Part model, mm, in its own coordinate system. A direction names the side the tool comes from. Coordinates: 2 decimals unless noted, no trailing zeros. Order: outer loops, then holes, each group sorted by start corner. A loop starts at its lowest first (then second) coordinate and runs counter-clockwise, first axis right, second up. Notation, with made-up numbers: (18.25, -23) - (59.25, -23) arc R12 ccw to (59.25, -12) - close; hole circle Ø3 at (16.25, 41.25). An arc over 180 degrees is marked (long way). Use a Markdown table: item, result. Add a question column.
1) Saw through at D-D on y = -12.5. List the corners of the cut face in (x, z).
2) Wall check: L1, parallel to Y at x = 0, z = 5.4; L2, parallel to Y at x = 0, z = 12; L3, parallel to Z at x = 1.5, y = 9.5. Give the ranges that are in metal, low to high. Write a range as [from, to].
3) Two-plate mould, pull along Z, no slides. Class faces 1 (the face through (-3, 7, 20)), 2 (the face through (8.873, -0.192, 13.098)), 3 (the face through (0, -9, 2)): +Z half, -Z half, draft (parallel to the pull), parting line (faces both ways), or undercut.
4) Saw through at B-B on x = 6. List the corners of the cut face in (y, z).
5) Saw through at A-A on y = 0. List the corners of the cut face in (x, z) (3 decimals), then the cut area to 4 significant figures.
6) Saw through at C-C on z = 3. List the corners of the cut face in (x, y), then the cut area to 3 significant figures.
7) Tool access for faces 4 (the face through (-2.981, -13.423, 4.986)), 5 (the face through (-8.873, 0.192, 13.098)), 6 (the face through (6.466, -2.681, 9.154)), 7 (the face through (9, 0, 4)): list every direction of +Z, -Z, +X, -X, +Y, -Y with a clear straight run to the whole face (end or side of a thin tool).
8) Drop flat-ended pins along their axis: P1, Ø12, axis at y = -13.5, z = 16.5, coming from the +X side; P2, Ø22, axis at x = 1, y = -6.5, coming from the +Z side; P3, Ø3, axis at y = -1, z = 7, coming from the +X side; P4, Ø6, axis at y = -9, z = 2.5, coming from the -X side. Give the stop position or say it passes through.
```python
from build123d import *

# Parameters (mm, degrees)
SKETCH1_R           = 13.75
BOSS_EXTRUDE1_DEPTH = 2
SKETCH2_R           = 8.5
BOSS_EXTRUDE2_DEPTH = 6
BOSS_EXTRUDE3_START = 4
SKETCH3_R           = 13.75
BOSS_EXTRUDE3_DEPTH = 2
SKETCH5_R           = 7
CUT_EXTRUDE2_DEPTH  = 37.5
BOSS_EXTRUDE4_START = 20
SKETCH6_R           = 8.875
SKETCH6_R_2         = 7
BOSS_EXTRUDE4_DEPTH = 14
CUT_EXTRUDE3_START  = 4
SKETCH9_R           = 0.25
CUT_EXTRUDE3_DEPTH  = 24.894892006
SKETCH10_R          = 19
BOSS_EXTRUDE5_DEPTH = 2
SKETCH11_R          = 7
CUT_EXTRUDE4_DEPTH  = 2
BOSS_EXTRUDE6_START = 2
SKETCH12_R          = 19
SKETCH12_R_2        = 17
BOSS_EXTRUDE6_DEPTH = 2


with BuildPart() as part:
    # Sketch1 → Boss-Extrude1 (new body)
    with BuildSketch(Plane.XY):
        Circle(SKETCH1_R)
    extrude(amount=BOSS_EXTRUDE1_DEPTH)

    # Sketch2 → Boss-Extrude2 (add)
    with BuildSketch(Plane.XY):
        Circle(SKETCH2_R)
    extrude(amount=BOSS_EXTRUDE2_DEPTH)

    # Sketch3 → Boss-Extrude3 (add)
    with BuildSketch(Plane.XY.offset(BOSS_EXTRUDE3_START)):
        Circle(SKETCH3_R)
    extrude(amount=BOSS_EXTRUDE3_DEPTH)

    # Sketch5 → Cut-Extrude2 (cut, symmetric)
    with BuildSketch(Plane.XY):
        Circle(SKETCH5_R)
    extrude(amount=CUT_EXTRUDE2_DEPTH, both=True, mode=Mode.SUBTRACT)

    # Sketch6 → Boss-Extrude4 (add)
    with BuildSketch(Plane.XY.offset(BOSS_EXTRUDE4_START)):
        Circle(SKETCH6_R)
        Circle(SKETCH6_R_2, mode=Mode.SUBTRACT)
    extrude(amount=-BOSS_EXTRUDE4_DEPTH)

    # Sketch9 → Cut-Extrude3 (cut, through all)
    with BuildSketch(Plane.XY.offset(CUT_EXTRUDE3_START)):
        with Locations((0, 9.75)):
            Circle(SKETCH9_R)
        with Locations((0, -9.75)):
            Circle(SKETCH9_R)
        with Locations(Location((0, 8.75, 0), (0, 0, 150.706355545))):
            Circle(SKETCH9_R)
        with Locations(Location((0, -8.75, 0), (0, 0, 209.293644455))):
            Circle(SKETCH9_R)
    extrude(amount=CUT_EXTRUDE3_DEPTH, mode=Mode.SUBTRACT)

    # Sketch10 → Boss-Extrude5 (add)
    with BuildSketch(Plane.XY):
        Circle(SKETCH10_R)
    extrude(amount=-BOSS_EXTRUDE5_DEPTH)

    # Sketch11 → Cut-Extrude4 (cut)
    with BuildSketch(Plane.XY):
        Circle(SKETCH11_R)
    extrude(amount=-CUT_EXTRUDE4_DEPTH, mode=Mode.SUBTRACT)

    # Sketch12 → Boss-Extrude6 (add)
    with BuildSketch(Plane.XY.offset(BOSS_EXTRUDE6_START)):
        Circle(SKETCH12_R)
        Circle(SKETCH12_R_2, mode=Mode.SUBTRACT)
    extrude(amount=-BOSS_EXTRUDE6_DEPTH)


solid = part.part
```
Results are:
| question | item | result |
|---|---|---|
| 1 | outline | (-14.31, -2) - (14.31, -2) - (14.31, 2) - (11.52, 2) - (11.52, 0) - (5.73, 0) - (5.73, 2) - (-5.73, 2) - (-5.73, 0) - (-11.52, 0) - (-11.52, 2) - (-14.31, 2) - close; (-5.73, 4) - (5.73, 4) - (5.73, 6) - (-5.73, 6) - close |
| 2 | L1 | [-13.75, -10], [-9.5, -9], [-8.5, -7], [7, 8.5], [9, 9.5], [10, 13.75] |
| 2 | L2 | [-8.5, -7], [7, 8.5] |
| 2 | L3 | [-2, 2], [4, 6] |
| 3 | face 1 | +Z half |
| 3 | face 2 | draft |
| 3 | face 3 | undercut |
| 4 | outline | (-18.03, -2) - (-3.61, -2) - (-3.61, 20) - (-6.54, 20) - (-6.54, 6) - (-12.37, 6) - (-12.37, 4) - (-6.02, 4) - (-6.02, 2) - (-12.37, 2) - (-12.37, 0) - (-15.91, 0) - (-15.91, 2) - (-18.03, 2) - close; (3.61, -2) - (18.03, -2) - (18.03, 2) - (15.91, 2) - (15.91, 0) - (12.37, 0) - (12.37, 2) - (6.02, 2) - (6.02, 4) - (12.37, 4) - (12.37, 6) - (6.54, 6) - (6.54, 20) - (3.61, 20) - close |
| 5 | outline | (-19, -2) - (-7, -2) - (-7, 20) - (-8.875, 20) - (-8.875, 6) - (-13.75, 6) - (-13.75, 4) - (-8.5, 4) - (-8.5, 2) - (-13.75, 2) - (-13.75, 0) - (-17, 0) - (-17, 2) - (-19, 2) - close; (7, -2) - (19, -2) - (19, 2) - (17, 2) - (17, 0) - (13.75, 0) - (13.75, 2) - (8.5, 2) - (8.5, 4) - (13.75, 4) - (13.75, 6) - (8.875, 6) - (8.875, 20) - (7, 20) - close |
| 5 | area | 168.5 mm2 |
| 6 | outline | circle Ø17 at (0, 0); hole circle Ø14 at (0, 0) |
| 6 | area | 73.0 mm2 |
| 7 | face 4 | +Z |
| 7 | face 5 | +Z, -X |
| 7 | face 6 | +Z, -Z |
| 7 | face 7 | none |
| 8 | P1 | x = 4.75 |
| 8 | P2 | z = 20 |
| 8 | P3 | x = 13.75 |
| 8 | P4 | x = -18.01 |
